Could you check a few things on this model? Use its own coordinates, in mm. A direction names the side the tool comes from. Round coordinates to 2 decimals unless told otherwise and drop trailing zeros. Order: outer loops, then holes, each group sorted by start corner. A loop starts at its lowest first (then second) coordinate and runs counter-clockwise, first axis right, second up. Notation, with made-up numbers: (35, -35) - (70, -35) arc R20 cw to (70, -8) - close; hole circle Ø5 at (78.5, 59). An arc over 180 degrees is marked (long way). Return JSON: item names as keys, results as strings. Group by question number.
Autodesk Inventor part; units mm, degrees
ref_plane "YZ Plane" through (0, 0, 0) normal (1, 0, 0) x (0, 1, 0)
ref_plane "XZ Plane" through (0, 0, 0) normal (0, 1, 0) x (-1, 0, 0)
ref_plane "XY Plane" through (0, 0, 0) normal (0, 0, 1) x (1, 0, 0)
sketch "Esquisse3" plane through (0, 0, 0) normal (1, 0, 0) x (0, 1, 0)
  line L0 (-7.2956, 0) -> (7.2956, 0)
  line L1 (5, 0) -> (5, 35)
  line L2 (5, 35) -> (4, 40)
  line L3 (4, 40) -> (0, 40)
  line L4 (0, 40) -> (0, 0)
  line L5 (0, 0) -> (5, 0)
  dimension "d1" = 5
  dimension "d2" = 4
  dimension "d3" = 5
  dimension "d4" = 80
revolve "Révolution1" add sketch "Esquisse3" angle 360 about axis through (0, -7.2956, 0) along (0, 1, 0)
sketch "Esquisse4" plane through (0, 5, 0) normal (0, 1, 0) x (1, 0, 0)
  point P0 (0, 0)
  point P1 (0, 0)
hole "Perçage1" at (0, 5, 0) direction (0, -1, 0) diameter 6.4 end through all counterbore diameter 12 counterbore depth 2
sketch "Esquisse5" plane through (0, 0, 0) normal (0, -1, 0) x (1, 0, 0)
  circle A0 centre (0, 30) radius 2
  point P0 (0, 0)
  dimension "d13" = 4
  dimension "d14" = 30
extrude "Extrusion1" add sketch "Esquisse5" along normal blind 2.8
chamfer "Chanfrein1" distance 1.5 angle 45 1 edges at (-2, -2.8, 30)
pattern_circular "Réseau circulaire1" count 3 over 360 about axis through (0, -10, 0) along (0, 1, 0) of "Extrusion1", "Chanfrein1"
properties part number "support_serrage_tourelle"
1) Will these pins go through, and if not, where does the flat tip stop? pin 1 (24 mm diameter, centred on x = -3.5, z = -6.5, fed in from -Y); pin 2 (7.5 mm diameter, centred on x = 0, z = 0, fed in from +Y); pin 3 (1 mm diameter, centred on y = -1, z = 16, fed in from -X); pin 4 (3 mm diameter, centred on y = -0.5, z = -13, fed in from +X).
2) For faces 1 (the cylindrical face through (1.947, 1.479, -2.539)), 2 (the cylindrical face through (24.507, -0.641, -16.352)), 3 (the flat face through (3, 3, 3)), which set-ups out of +Z, -Z, +X, -X, +Y, -Y let a thin tool reach every point of the face, with its end or its side?
3) If I drill on line 1 along X through (y, z) = (3.5, 0); line 2 along X through (y, z) = (0.9, 0); line 3 along Y through (x, z) = (-1.5, -26), over which ranges is the centre line in solid material (lowest first)? Write a range as from..to.
4) We'd pull the mould along X, two halves only. Please class faces 4 (the flat face through (-7, 5, 0)), 5 (the cylindrical face through (0, -1, 32)), 6 (the cylindrical face through (-26, -1, -13)), 7 (the cylindrical face through (0, 4, -6)): +X half, -X half, draft (parallel to the pull), parting line (faces both ways), or undercut.
5) I want a section at A-A, the plane z = 0. List the corners of the cut face in (x, y) for me, plus the area to 3 significant figures.
6) I want a section at B-B, the plane y = 1.25. List the corners of the cut face in (x, z) for me, plus the area to 3 significant figures.
Outcome:
{
 "1": {"pin 1": "y = 0", "pin 2": "y = 3", "pin 3": "through", "pin 4": "x = 38.29"},
 "2": {"face 1": "+Y, -Y", "face 2": "-Y", "face 3": "+Y"},
 "3": {"line 1": "-40..-6, 6..40", "line 2": "-40..-3.2, 3.2..40", "line 3": "0..5"},
 "4": {"face 4": "draft", "face 5": "parting line", "face 6": "undercut", "face 7": "undercut"},
 "5": {"outline": "(-40, 0) - (-3.2, 0) - (-3.2, 3) - (-6, 3) - (-6, 5) - (-35, 5) - (-40, 4) - close; (3.2, 0) - (40, 0) - (40, 4) - (35, 5) - (6, 5) - (6, 3) - (3.2, 3) - close", "area": "352 mm^2"},
 "6": {"outline": "circle Ø80 at (0, 0); hole circle Ø6.4 at (0, 0)", "area": "4,990 mm^2"}
}
